For this review, use the dimensioned drawing (mm, ordinates from the lowest corner) and the shaded views. A direction names the side the tool comes from. Round coordinates to 2 decimals unless told otherwise and drop trailing zeros. Loops run counter-clockwise (first coordinate to the right, second up) from the corner with the lowest first, then second, coordinate; pieces in that order, holes last. Notation, with made-up numbers: M -20.5,65 L 33.5,65 A18 cw 33.5,86 Z; hole C -28.5,24 d10. An arc over 180 degrees is marked long. Answer as a JSON object with one key per item and string values. Group by question number.
Item 1: Consider section B-B (x = 11.5). Give the boundary of the cut face in (y, z), and give its area (3 significant figures).
Item 2: Consider section C-C (z = 3.75). Give the boundary of the cut face in (x, y).
Item 3: Tool access review of the marked faces 1 and 2: name each direction out of +Z, -Z, +X, -X, +Y, -Y from which nothing blocks a thin tool from reaching the whole face with its end or side.
Item 4: Insertion check: P1, Ø6, axis at x = 11.5, z = 11.5, coming from the +Y side; P2, Ø12, axis at x = 16.5, y = 19, coming from the -Z side. Each pin has a flat end and moves straight along its axis. Give the tip position at first contact, or say it passes through.
Item 5: Consider section A-A (z = 6.35). Give the boundary of the cut face in (x, y), and give its area (3 significant figures).
Item 6: To check wall thickness, follow line 1 (Y direction, x = 17.25, z = 11). State the ranges of the line that lie inside material, in increasing order.
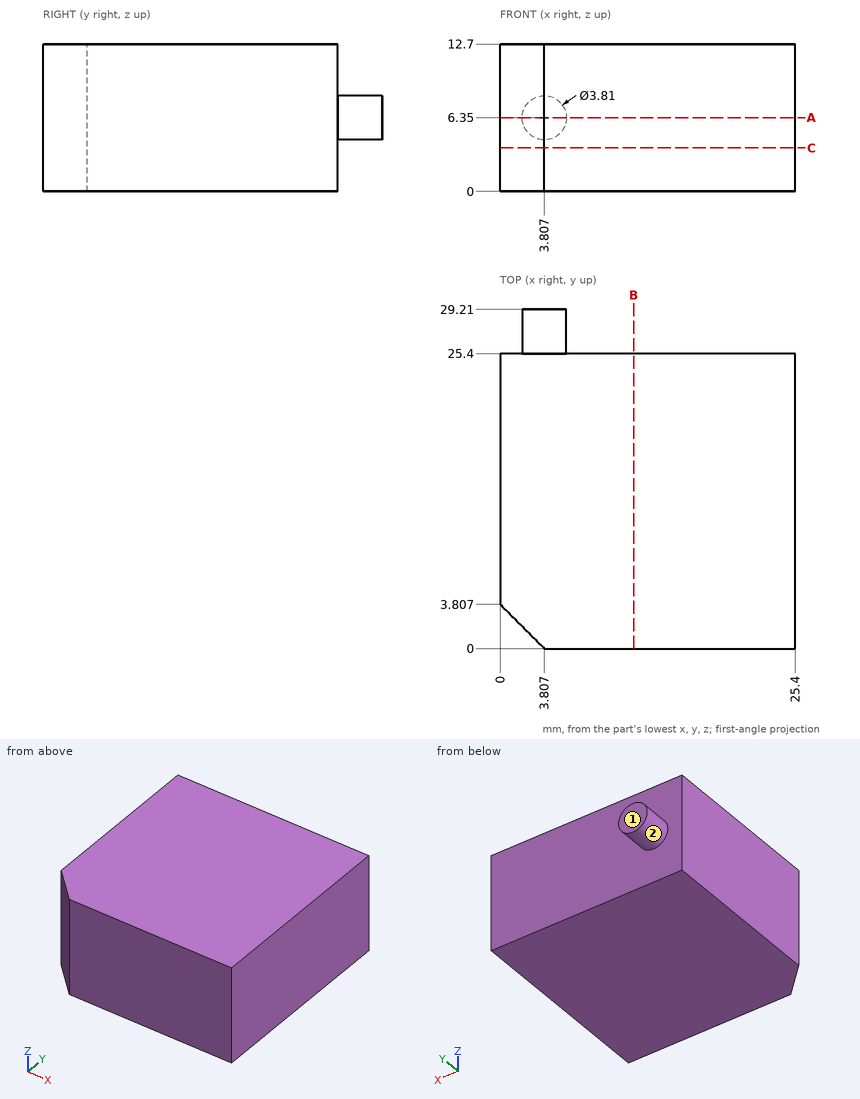
Geometry results:
{
 "1": {"outline": "M 0,0 L 25.4,0 L 25.4,12.7 L 0,12.7 Z", "area": "323 mm^2"},
 "2": {"outline": "M 0,3.81 L 3.81,0 L 25.4,0 L 25.4,25.4 L 0,25.4 Z"},
 "3": {"face 1": "+Z, -Z, +X, -X, +Y", "face 2": "+Y"},
 "4": {"P1": "stops at y = 25.4", "P2": "stops at z = 0"},
 "5": {"outline": "M 0,3.81 L 3.81,0 L 25.4,0 L 25.4,25.4 L 5.71,25.4 L 5.71,29.21 L 1.9,29.21 L 1.9,25.4 L 0,25.4 Z", "area": "652 mm^2"},
 "6": {"line 1": "y = 0 to 25.4"}
}
